from build123d import *

# Parameters (mm, degrees)
F0_R     = 15
F1_DEPTH = 124
F3_DEPTH = 40
F4_R     = 15
F5_DEPTH = 45
F7_DEPTH = 100
F8_R     = 150
F8_R_2   = 15
F9_DEPTH = 120


with BuildPart() as f1:
    # F0 (on Right) → F1 (new body)
    with BuildSketch(Plane.YZ):
        Polygon((-55.507882, 234.50625), (-150.260191, 139.753941), (-224.506403, 65.507729), (-170, 11.001326), (-170, -110.50625), (-144.782609, -110.50625), (-144.782609, -234.50625), (144.782609, -234.50625), (144.782609, -110.50625), (170, -110.50625), (170, 11.001326), (224.506403, 65.507729), (150.260191, 139.753941), (55.507882, 234.50625), align=None)
        with Locations((0, -10.50625)):
            Circle(F0_R, mode=Mode.SUBTRACT)
    extrude(amount=F1_DEPTH)

    # F2 (on face) → F3 (join)
    with BuildSketch(Plane.YZ.offset(124)):
        Polygon((0, 224.50625), (-51.3657463763, 224.50625), (-158, 117.8719963763), (-158, -100.50625), (-134.782609, -100.50625), (-134.782609, -224.50625), (0, -224.50625), (134.782609, -224.50625), (134.782609, -100.50625), (158, -100.50625), (158, 117.8719963763), (51.3657463763, 224.50625), align=None)
        with BuildLine():
            ThreePointArc((15, -10.50625), (-10.6066017178, -21.1128517178), (0, 4.49375))
            ThreePointArc((0, 4.49375), (10.6066017178, 0.1003517178), (15, -10.50625))
        make_face(mode=Mode.SUBTRACT)
    extrude(amount=F3_DEPTH)

    # F4 (on face) → F5 (join)
    with BuildSketch(Plane(origin=(0, 0, 0), x_dir=(0, -1, 0), z_dir=(-1, 0, 0))):
        Polygon((134.782609, -100.50625), (158, -100.50625), (158, 117.8719963763), (51.3657463763, 224.50625), (0, 224.50625), (-51.3657463763, 224.50625), (-158, 117.8719963763), (-158, -100.50625), (-134.782609, -100.50625), (-134.782609, -224.50625), (0, -224.50625), (134.782609, -224.50625), align=None)
        with Locations((0, -10.50625)):
            Circle(F4_R, mode=Mode.SUBTRACT)
    extrude(amount=F5_DEPTH)

    # F6 (on face) → F7 (join)
    with BuildSketch(Plane(origin=(0, -145.007066, 145.007066), x_dir=(1, 0, 0), z_dir=(0, -0.7071067812, 0.7071067812))):
        with BuildLine():
            ThreePointArc((124, -61.8555966032), (139.2050840295, -36.5086726323), (144.5, -7.4290405851))
            ThreePointArc((144.5, -7.4290405851), (139.2050840295, 21.6505914621), (124, 46.9975154331))
            Line((124, 46.9975154331), (124, 29.1769698504))
            ThreePointArc((124, 29.1769698504), (131.4550214167, 11.5446253759), (134, -7.4290405851))
            ThreePointArc((134, -7.4290405851), (131.4550214167, -26.4027065461), (124, -44.0350510205))
            Line((124, -44.0350510205), (124, -61.8555966032))
        make_face()
        with BuildLine():
            ThreePointArc((0, -61.8555966032), (62, -89.9290405851), (124, -61.8555966032))
            Line((124, -61.8555966032), (124, -44.0350510205))
            ThreePointArc((124, -44.0350510205), (62, -79.4290405851), (0, -44.0350510205))
            Line((0, -44.0350510205), (0, -61.8555966033))
        make_face()
        with BuildLine():
            Line((0, 29.1769698504), (0, 46.9975154331))
            ThreePointArc((0, 46.9975154331), (-20.5, -7.4290405851), (0, -61.8555966032))
            Line((0, -61.8555966033), (0, -44.0350510205))
            ThreePointArc((0, -44.0350510205), (-10, -7.4290405851), (0, 29.1769698504))
        make_face()
    extrude(amount=-F7_DEPTH)

    # F8 (on face) → F9 (cut)
    with BuildSketch(Plane.YZ.offset(164)):
        with Locations((0, -10.50625)):
            Circle(F8_R)
        with Locations((0, -10.50625)):
            Circle(F8_R_2, mode=Mode.SUBTRACT)
    extrude(amount=-F9_DEPTH, mode=Mode.SUBTRACT)


solid = f1.part
Input: part model. Units: mm. Frame: model coordinates. A direction names the side the tool comes from. Coordinates: 2 decimals unless noted, no trailing zeros. Write each loop counter-clockwise with the first axis right and the second up, starting at its lowest first coordinate (ties: lowest second). Pieces come first, ordered by that corner, then holes. Notation, with made-up numbers: M 29.5,7.5 L 87.5,7.5 A10 cw 87.5,15.5 Z; hole C -4.5,68.25 d1. An arc over 180 degrees is marked long. Answer as a JSON object with one key per item and string values. Group by question number.
(1) Section D-D on y = 126.5. Output: boundary loops of the cut face in (x, z).
(2) Mould query, pull axis Y, two halves, no side actions, for faces 4 (the face through (-22, 158, 10)), 5 (the face through (-18.686, -157.374, 122.535)), 6 (the face through (61, -198, 39)). Classes: pulls with the +Y half, pulls with the -Y half, needs draft (parallel to the pull), parting line crosses it, or undercut.
(3) Section C-C on x = 90.5. Output: boundary loops of the cut face in (y, z), plus the area to 3 significant figures.
(4) Contact query for flat-ended pins moving along their axis: P1, Ø10, axis at x = 44, y = 148, coming from the -Z side; P2, Ø4, axis at x = 94.5, z = -85, coming from the +Y side; P3, Ø3.5, axis at x = -4, z = 108, coming from the -Y side; P4, Ø5, axis at x = 10.5, z = 112, coming from the -Y side. Output: stop coordinate, or through.
(5) Section A-A on y = 0. Output: boundary loops of the cut face in (x, z).
(6) Set-up query: faces 1 (the face through (61, 144.783, -173)), 2 (the face through (-10, -145.7, 134.5)), 3 (the face through (44, -2, -42)). Return all of +Z, -Z, +X, -X, +Y, -Y with unobstructed straight access to the full face (end or side cutting, diameter ignored); none if empty.
(7) Section B-B on z = -175.5. Output: boundary loops of the cut face in (x, y), plus the area to 3 significant figures.
(8) Ray query, line 1 along Z through (x, y) = (70, 0); line 2 along Z through (x, y) = (-34, 0); line 3 along X through (y, z) = (126, -45). Return the intervals inside material, ascending. Write a range as [from, to].
Result set:
{
 "1": {"outline": "M -45,-224.51 L 0,-224.51 L 0,-234.51 L 124,-234.51 L 124,-224.51 L 164,-224.51 L 164,-91.11 L 44,-91.11 L 44,70.1 L 164,70.1 L 164,149.37 L 124,149.37 L 124,163.51 L 0,163.51 L 0,149.37 L -45,149.37 Z"},
 "2": {"face 4": "pulls with the +Y half", "face 5": "undercut", "face 6": "pulls with the -Y half"},
 "3": {"outline": "M -224.51,65.51 L -170,11 L -170,-110.51 L -144.78,-110.51 L -144.78,-234.51 L 144.78,-234.51 L 144.78,-110.51 L 170,-110.51 L 170,11 L 224.51,65.51 L 55.51,234.51 L -55.51,234.51 Z; hole C 0,-10.51 d300", "area": "75,400 mm2"},
 "4": {"P1": "stops at z = -234.51", "P2": "stops at y = 170", "P3": "stops at y = -183.76", "P4": "stops at y = -180.51"},
 "5": {"outline": "M -45,-224.51 L 0,-224.51 L 0,-234.51 L 124,-234.51 L 124,-224.51 L 164,-224.51 L 164,-160.51 L 44,-160.51 L 44,-25.51 L -45,-25.51 Z; M -45,4.49 L 44,4.49 L 44,139.49 L 164,139.49 L 164,224.51 L 124,224.51 L 124,234.51 L 0,234.51 L 0,224.51 L -45,224.51 Z"},
 "6": {"face 1": "-Z, +X, -X, +Y", "face 2": "none", "face 3": "+X"},
 "7": {"outline": "M -45,-134.78 L 0,-134.78 L 0,-144.78 L 124,-144.78 L 124,-134.78 L 164,-134.78 L 164,134.78 L 124,134.78 L 124,144.78 L 0,144.78 L 0,134.78 L -45,134.78 Z", "area": "58,800 mm2"},
 "8": {"line 1": "z = [-234.51, -160.51], [139.49, 234.51]", "line 2": "z = [-224.51, -25.51], [4.49, 224.51]", "line 3": "x = [-45, 44]"}
}
